from build123d import *

# Parameters (mm, degrees)
SKETCH1_W           = 38
SKETCH1_H           = 23
BOSS_EXTRUDE1_DEPTH = 1.5875
CUT_EXTRUDE1_REACH  = 24.266
SKETCH2_R           = 1.25


with BuildPart() as part:
    # Sketch1 → Boss-Extrude1 (new body)
    with BuildSketch(Plane(origin=(0, 0, 0), x_dir=(1, 0, 0), z_dir=(0, 1, 0))):
        Rectangle(SKETCH1_W, SKETCH1_H)
    extrude(amount=BOSS_EXTRUDE1_DEPTH)

    # Sketch2 → Cut-Extrude1 (cut, up to next)
    with BuildSketch(Plane(origin=(0, 1.5875, 0), x_dir=(1, 0, 0), z_dir=(0, 1, 0)), mode=Mode.PRIVATE) as cut_extrude1_sk1:
        with BuildLine():
            Line((-19, 11.5), (-19, 8.95))
            ThreePointArc((-19, 8.95), (-18.253122292, 10.753122292), (-16.45, 11.5))
            Line((-16.45, 11.5), (-19, 11.5))
        make_face()
    cut_extrude1_tool1 = extrude(cut_extrude1_sk1.sketch, amount=-CUT_EXTRUDE1_REACH, mode=Mode.PRIVATE) & part.part
    # Sketch2 → Cut-Extrude1 (cut, up to next)
    with BuildSketch(Plane(origin=(0, 1.5875, 0), x_dir=(1, 0, 0), z_dir=(0, 1, 0)), mode=Mode.PRIVATE) as cut_extrude1_sk2:
        with Locations(Location((-16.45, 8.95, 0), (0, 0, 270))):
            Circle(SKETCH2_R)
    cut_extrude1_tool2 = extrude(cut_extrude1_sk2.sketch, amount=-CUT_EXTRUDE1_REACH, mode=Mode.PRIVATE) & part.part
    # Sketch2 → Cut-Extrude1 (cut, up to next)
    with BuildSketch(Plane(origin=(0, 1.5875, 0), x_dir=(1, 0, 0), z_dir=(0, 1, 0)), mode=Mode.PRIVATE) as cut_extrude1_sk3:
        with BuildLine():
            Line((-14.9, 6.4), (-16.45, 6.4))
            ThreePointArc((-16.45, 6.4), (-18.253122292, 7.146877708), (-19, 8.95))
            Line((-19, 8.95), (-19, -8.95))
            ThreePointArc((-19, -8.95), (-18.253122292, -7.146877708), (-16.45, -6.4))
            Line((-16.45, -6.4), (-14.9, -6.4))
            ThreePointArc((-14.9, -6.4), (-14.192893219, -6.107106781), (-13.9, -5.4))
            Line((-13.9, -5.4), (-13.9, 5.4))
            ThreePointArc((-13.9, 5.4), (-14.192893219, 6.107106781), (-14.9, 6.4))
        make_face()
    cut_extrude1_tool3 = extrude(cut_extrude1_sk3.sketch, amount=-CUT_EXTRUDE1_REACH, mode=Mode.PRIVATE) & part.part
    # Sketch2 → Cut-Extrude1 (cut, up to next)
    with BuildSketch(Plane(origin=(0, 1.5875, 0), x_dir=(1, 0, 0), z_dir=(0, 1, 0)), mode=Mode.PRIVATE) as cut_extrude1_sk4:
        with BuildLine():
            ThreePointArc((-16.45, -11.5), (-18.253122292, -10.753122292), (-19, -8.95))
            Line((-19, -8.95), (-19, -11.5))
            Line((-19, -11.5), (-16.45, -11.5))
        make_face()
    cut_extrude1_tool4 = extrude(cut_extrude1_sk4.sketch, amount=-CUT_EXTRUDE1_REACH, mode=Mode.PRIVATE) & part.part
    # Sketch2 → Cut-Extrude1 (cut, up to next)
    with BuildSketch(Plane(origin=(0, 1.5875, 0), x_dir=(1, 0, 0), z_dir=(0, 1, 0)), mode=Mode.PRIVATE) as cut_extrude1_sk5:
        with Locations(Location((-16.45, -8.95, 0), (0, 0, 270))):
            Circle(SKETCH2_R)
    cut_extrude1_tool5 = extrude(cut_extrude1_sk5.sketch, amount=-CUT_EXTRUDE1_REACH, mode=Mode.PRIVATE) & part.part
    # Sketch2 → Cut-Extrude1 (cut, up to next)
    with BuildSketch(Plane(origin=(0, 1.5875, 0), x_dir=(1, 0, 0), z_dir=(0, 1, 0)), mode=Mode.PRIVATE) as cut_extrude1_sk6:
        with Locations(Location((16.45, -8.95, 0), (0, 0, 270))):
            Circle(SKETCH2_R)
    cut_extrude1_tool6 = extrude(cut_extrude1_sk6.sketch, amount=-CUT_EXTRUDE1_REACH, mode=Mode.PRIVATE) & part.part
    # Sketch2 → Cut-Extrude1 (cut, up to next)
    with BuildSketch(Plane(origin=(0, 1.5875, 0), x_dir=(1, 0, 0), z_dir=(0, 1, 0)), mode=Mode.PRIVATE) as cut_extrude1_sk7:
        with BuildLine():
            ThreePointArc((19, -8.95), (18.253122304, -10.75312228), (16.450000035, -11.5))
            Line((16.450000035, -11.5), (19, -11.5))
            Line((19, -11.5), (19, -8.95))
        make_face()
    cut_extrude1_tool7 = extrude(cut_extrude1_sk7.sketch, amount=-CUT_EXTRUDE1_REACH, mode=Mode.PRIVATE) & part.part
    # Sketch2 → Cut-Extrude1 (cut, up to next)
    with BuildSketch(Plane(origin=(0, 1.5875, 0), x_dir=(1, 0, 0), z_dir=(0, 1, 0)), mode=Mode.PRIVATE) as cut_extrude1_sk8:
        with BuildLine():
            Line((19, -8.95), (19, 8.95))
            ThreePointArc((19, 8.95), (18.253122292, 7.146877708), (16.45, 6.4))
            Line((16.45, 6.4), (14.9, 6.4))
            ThreePointArc((14.9, 6.4), (14.192893219, 6.107106781), (13.9, 5.4))
            Line((13.9, 5.4), (13.9, -5.4))
            ThreePointArc((13.9, -5.4), (14.192893219, -6.107106781), (14.9, -6.4))
            Line((14.9, -6.4), (16.45, -6.4))
            ThreePointArc((16.45, -6.4), (18.253122292, -7.146877708), (19, -8.95))
        make_face()
    cut_extrude1_tool8 = extrude(cut_extrude1_sk8.sketch, amount=-CUT_EXTRUDE1_REACH, mode=Mode.PRIVATE) & part.part
    # Sketch2 → Cut-Extrude1 (cut, up to next)
    with BuildSketch(Plane(origin=(0, 1.5875, 0), x_dir=(1, 0, 0), z_dir=(0, 1, 0)), mode=Mode.PRIVATE) as cut_extrude1_sk9:
        with BuildLine():
            Line((19, 11.5), (16.45, 11.5))
            ThreePointArc((16.45, 11.5), (18.253122292, 10.753122292), (19, 8.95))
            Line((19, 8.95), (19, 11.5))
        make_face()
    cut_extrude1_tool9 = extrude(cut_extrude1_sk9.sketch, amount=-CUT_EXTRUDE1_REACH, mode=Mode.PRIVATE) & part.part
    # Sketch2 → Cut-Extrude1 (cut, up to next)
    with BuildSketch(Plane(origin=(0, 1.5875, 0), x_dir=(1, 0, 0), z_dir=(0, 1, 0)), mode=Mode.PRIVATE) as cut_extrude1_sk10:
        with Locations(Location((16.45, 8.95, 0), (0, 0, 270))):
            Circle(SKETCH2_R)
    cut_extrude1_tool10 = extrude(cut_extrude1_sk10.sketch, amount=-CUT_EXTRUDE1_REACH, mode=Mode.PRIVATE) & part.part
    add(cut_extrude1_tool1.solids().sort_by_distance((-18.430412, 1.5875, -10.930412))[0], mode=Mode.SUBTRACT)
    add(cut_extrude1_tool2.solids().sort_by_distance((-16.45, 1.5875, -8.95))[0], mode=Mode.SUBTRACT)
    add(cut_extrude1_tool3.solids().sort_by_distance((-16.546475, 1.5875, 0))[0], mode=Mode.SUBTRACT)
    add(cut_extrude1_tool4.solids().sort_by_distance((-18.430412, 1.5875, 10.930412))[0], mode=Mode.SUBTRACT)
    add(cut_extrude1_tool5.solids().sort_by_distance((-16.45, 1.5875, 8.95))[0], mode=Mode.SUBTRACT)
    add(cut_extrude1_tool6.solids().sort_by_distance((16.45, 1.5875, 8.95))[0], mode=Mode.SUBTRACT)
    add(cut_extrude1_tool7.solids().sort_by_distance((18.430412, 1.5875, 10.930412))[0], mode=Mode.SUBTRACT)
    add(cut_extrude1_tool8.solids().sort_by_distance((16.546475, 1.5875, 0))[0], mode=Mode.SUBTRACT)
    add(cut_extrude1_tool9.solids().sort_by_distance((18.430412, 1.5875, -10.930412))[0], mode=Mode.SUBTRACT)
    add(cut_extrude1_tool10.solids().sort_by_distance((16.45, 1.5875, -8.95))[0], mode=Mode.SUBTRACT)


solid = part.part
Design review of the part built by this model. Coordinates are the model's own, in mm. A direction names the side the tool comes from. Coordinates: 2 decimals unless noted, no trailing zeros. Loops run counter-clockwise (first coordinate to the right, second up) from the corner with the lowest first, then second, coordinate; pieces in that order, holes last. Notation, with made-up numbers: M -28,9 L -18,9 A22 cw -18,47 Z; hole C 51,16.25 d2. An arc over 180 degrees is marked long. Answer as CSV lines item,"result".
Item 1: Add section B-B on z = -8.5. State the section outline as (x, y) points, plus the area to 3 significant figures.
Answer list:
outline,"M -18.96,0 L -17.62,0 L -17.62,1.59 L -18.96,1.59 Z; M -15.28,0 L 15.28,0 L 15.28,1.59 L -15.28,1.59 Z; M 17.62,0 L 18.96,0 L 18.96,1.59 L 17.62,1.59 Z"
area,"52.8 mm²"
Item 2: The part is to be moulded in two halves that separate along X. For faces 1 (the face through (16, 1, -6.4)), 2 (the face through (-17.67, 0.8, -9.22)), 3 (the face through (-14.185, 0.805, -6.099)), 4 (the face through (14.201, 0.805, -6.115)), say which applies: pulls with the +X half, pulls with the -X half, needs draft (parallel to the pull), parting line crosses it, or undercut.
Answer list:
face 1,"needs draft"
face 2,"undercut"
face 3,"pulls with the -X half"
face 4,"pulls with the +X half"
Item 3: For probe 1 along X at (y, z) = (0.4, 8.95); probe 2 along X at (y, z) = (1.1, -8); probe 3 along Z at (x, y) = (-15.5, 0.95), list the stretches that pass through material, from the lowest coordinate up.
Answer list:
probe 1,"-19 to -17.7, -15.2 to 15.2, 17.7 to 19"
probe 2,"-18.82 to -17.26, -15.64 to 15.64, 17.26 to 18.82"
probe 3,"-11.5 to -9.76, -8.14 to -6.4, 6.4 to 8.14, 9.76 to 11.5"
Item 4: Machinability: for faces 5 (the face through (0, 1, 11.5)), 6 (the face through (13.9, 1, 0)), 7 (the face through (-16, 1, -6.4)), which of the approach directions +Z, -Z, +X, -X, +Y, -Y give a long, thin tool a straight path to every point of the face, cutting with its end or side? Answer none if there is none.
Answer list:
face 5,"+Z, +X, -X, +Y, -Y"
face 6,"+X, +Y, -Y"
face 7,"-X, +Y, -Y"
Item 5: For P1, Ø2, axis at x = 16.45, z = 8.95, coming from the +Y side; P2, Ø0.8, axis at y = 0.5, z = -1, coming from the -X side, all flat-tipped, find the tip position at first contact; note any pin that passes through.
Answer list:
P1,"through"
P2,"x = -13.9"
Item 6: Add section A-A on y = 1.25. State the section outline as (x, z) points.
Answer list:
outline,"M -16.45,-11.5 L 16.45,-11.5 A2.55 ccw 16.45,-6.4 L 14.9,-6.4 A1 cw 13.9,-5.4 L 13.9,5.4 A1 cw 14.9,6.4 L 16.45,6.4 A2.55 ccw 16.45,11.5 L -16.45,11.5 A2.55 ccw -16.45,6.4 L -14.9,6.4 A1 cw -13.9,5.4 L -13.9,-5.4 A1 cw -14.9,-6.4 L -16.45,-6.4 A2.55 ccw Z; hole C -16.45,-8.95 d2.5; hole C -16.45,8.95 d2.5; hole C 16.45,-8.95 d2.5; hole C 16.45,8.95 d2.5"
Item 7: Add section C-C on z = 0. State the section outline as (x, y) points.
Answer list:
outline,"M -13.9,0 L 13.9,0 L 13.9,1.59 L -13.9,1.59 Z"
